Verification items for the finished model (mm, model axes). A direction names the side the tool comes from. Coordinates: 2 decimals unless noted, no trailing zeros. Write each loop counter-clockwise with the first axis right and the second up, starting at its lowest first coordinate (ties: lowest second). Pieces come first, ordered by that corner, then holes. Notation, with made-up numbers: (-12, -36.5) -> (23, -36.5) arc R16 ccw to (23, -23.5) -> close; hole circle Ø6 at (74.5, -15.5). An arc over 180 degrees is marked (long way). Answer in a Markdown table with one row per item.
```python
from build123d import *

# Parameters (mm, degrees)
SKETCH001_R     = 2.75
PAD001_DEPTH    = 17
POCKET_DEPTH    = 12
SKETCH002_R     = 2.75
POCKET001_DEPTH = 5.001
SKETCH004_R     = 3.75
SKETCH004_R_2   = 2.75
PAD_DEPTH       = 0.5
PAD002_DEPTH    = 14
SKETCH006_R     = 6
POCKET002_DEPTH = 11


with BuildPart() as part:
    # Sketch001 → Pad001 (new body)
    with BuildSketch(Plane.XY.offset(6)):
        Polygon((15, -30), (-20, -30), (-20, 20), (30, 20), (30, -15), align=None)
        with Locations((-10, -20)):
            Circle(SKETCH001_R, mode=Mode.SUBTRACT)
        with Locations((20, 10)):
            Circle(SKETCH001_R, mode=Mode.SUBTRACT)
    extrude(amount=PAD001_DEPTH)

    # Sketch (on Face8 of Pad001) → Pocket (cut)
    with BuildSketch(Plane(origin=(0, 0, 6), x_dir=(1, 0, 0), z_dir=(0, 0, -1))):
        Polygon((15, 30), (3, 30), (3, 16), (16, 3), (30, 3), (30, 15), align=None)
    extrude(amount=-POCKET_DEPTH, mode=Mode.SUBTRACT)

    # Sketch002 (on Face2 of Pocket) → Pocket001 (cut, through all)
    with BuildSketch(Plane(origin=(0, 0, 18), x_dir=(1, 0, 0), z_dir=(0, 0, -1))):
        with Locations((18, 18)):
            Circle(SKETCH002_R)
    extrude(amount=-POCKET001_DEPTH, mode=Mode.SUBTRACT)

    # Sketch004 (on Face2 of Pocket001) → Pad (join)
    with BuildSketch(Plane(origin=(0, 0, 18), x_dir=(1, 0, 0), z_dir=(0, 0, -1))):
        with Locations((18, 18)):
            Circle(SKETCH004_R)
        with Locations((18, 18)):
            Circle(SKETCH004_R_2, mode=Mode.SUBTRACT)
    extrude(amount=PAD_DEPTH)

    # Sketch005 (on Face4 of Pad) → Pad002 (join)
    with BuildSketch(Plane(origin=(0, 0, 6), x_dir=(1, 0, 0), z_dir=(0, 0, -1))):
        Polygon((3, 16), (16, 3), (30, 3), (30, 0), (0, 0), (0, 30), (3, 30), align=None)
    extrude(amount=PAD002_DEPTH)

    # Sketch006 (on Face5 of Pad002) → Pocket002 (cut)
    with BuildSketch(Plane.XY.offset(23)):
        with Locations((20, 10)):
            Circle(SKETCH006_R)
        with Locations((-10, -20)):
            Circle(SKETCH006_R)
    extrude(amount=-POCKET002_DEPTH, mode=Mode.SUBTRACT)


solid = part.part
```
1. Mould release check, pull along X, two halves, no side actions. Record for faces 1 (the cylindrical face through (17.19, -14.34, 17.75)), 2 (the flat face through (30, 6, 15)), 3 (the flat face through (8, -8, -8)): released by +X, released by -X, zero draft, split by the parting line, or undercut.
Geometry says:
| item | result |
|---|---|
| face 1 | undercut |
| face 2 | released by +X |
| face 3 | zero draft |
2. Tool access check on faces 4 (the flat face through (17, -21, 17.5)), 5 (the flat face through (15, 0, -1)), 6 (the flat face through (16, -14, 18)), 7 (the cylindrical face through (22.769, 4.677, 17.577)). Record the directions out of +Z, -Z, +X, -X, +Y, -Y that give a thin tool (end or side, any length) a straight path to the whole face; none if there is none.
Geometry says:
| item | result |
|---|---|
| face 4 | -Z, +X, -Y |
| face 5 | -Z, +X, -X, +Y |
| face 6 | -Z |
| face 7 | +Z |
3. Section check B-B, the plane y = 10. Record the boundary of the cut face in (x, z).
Geometry says:
| item | result |
|---|---|
| outline | (-20, 6) -> (17.25, 6) -> (17.25, 12) -> (14, 12) -> (14, 23) -> (-20, 23) -> close; (22.75, 6) -> (30, 6) -> (30, 23) -> (26, 23) -> (26, 12) -> (22.75, 12) -> close |
4. Section check D-D, the plane y = -18. Record the boundary of the cut face in (x, z), plus the area to 3 significant figures.
Geometry says:
| item | result |
|---|---|
| outline | (-20, 6) -> (-11.89, 6) -> (-11.89, 12) -> (-15.66, 12) -> (-15.66, 23) -> (-20, 23) -> close; (-8.11, 6) -> (0, 6) -> (0, -8) -> (3, -8) -> (3, 18) -> (14.25, 18) -> (14.25, 17.5) -> (15.25, 17.5) -> (15.25, 23) -> (-4.34, 23) -> (-4.34, 12) -> (-8.11, 12) -> close; (20.75, 17.5) -> (21.75, 17.5) -> (21.75, 18) -> (27, 18) -> (27, 23) -> (20.75, 23) -> close |
| area | 379 mm^2 |
5. Section check C-C, the plane z = 13.5. Record the boundary of the cut face in (x, y), plus the area to 3 significant figures.
Geometry says:
| item | result |
|---|---|
| outline | (-20, -30) -> (3, -30) -> (3, -16) -> (16, -3) -> (30, -3) -> (30, 20) -> (-20, 20) -> close; hole circle Ø12 at (-10, -20); hole circle Ø12 at (20, 10) |
| area | 1,630 mm^2 |
6. Depth check by flat-ended pin: P1, Ø8, axis at x = 14.5, y = -20, coming from the -Z side; P2, Ø3.5, axis at x = 18, y = -18, coming from the -Z side; P3, Ø15, axis at x = 11.5, y = -9.5, coming from the -Z side; P4, Ø7, axis at y = -10.5, z = -1, coming from the -X side. Enter the tip coordinate at first touch or a pass-through.
Geometry says:
| item | result |
|---|---|
| P1 | z = 17.5 |
| P2 | through |
| P3 | z = -8 |
| P4 | x = 0 |
7. Thickness scan on line 1 (X direction, y = -18, z = 17.9); line 2 (X direction, y = -18, z = 21); line 3 (Y direction, x = 20, z = 20.75). Record the ranges inside material, lowest first. Write a range as from..to.
Geometry says:
| item | result |
|---|---|
| line 1 | -20..-15.66, -4.34..3, 14.25..15.25, 20.75..21.75 |
| line 2 | -20..-15.66, -4.34..15.25, 20.75..27 |
| line 3 | -25..-19.89, -16.11..4, 16..20 |
8. Section check A-A, the plane x = -10. Record the boundary of the cut face in (y, z), plus the area to 3 significant figures.
Geometry says:
| item | result |
|---|---|
| outline | (-30, 6) -> (-22.75, 6) -> (-22.75, 12) -> (-26, 12) -> (-26, 23) -> (-30, 23) -> close; (-17.25, 6) -> (20, 6) -> (20, 23) -> (-14, 23) -> (-14, 12) -> (-17.25, 12) -> close |
| area | 685 mm^2 |
